The listing builds one solid part. Answer for the finished solid, in the listing's coordinates (mm). Coordinates: 2 decimals unless noted, no trailing zeros.
(1) For a pull along Y with two mould halves and no side action, classify faces 1 (the cylindrical face through (1.359, -1.683, 49.002)), 2 (the flat face through (0, 0, 0)) as +Y half, -Y half, draft (parallel to the pull), parting line (faces both ways), or undercut.
(2) Given P1, Ø4, axis at x = -9, z = 27.5, coming from the +Y side; P2, Ø1.6, axis at x = -1.905, y = -2.54, coming from the +Z side; P3, Ø1.5, axis at y = 18, z = 10.5, coming from the +X side, each flat-ended and moving along its own axis, determine where each tip first touches the part or whether it passes through.
(3) Straight lines are drawn through the part: line 1 (X direction, y = -2.54, z = 49); line 2 (X direction, y = -2, z = 48); line 3 (Y direction, x = 17, z = 12). For each, find the intervals that lie inside material, in ascending order.
from build123d import *

# Parameters (mm, degrees)
F4_D     = 2.032
F4_DEPTH = 3.81
F4_START = 13.0290755
F4_TIP   = 0.6104743889
F5_DEPTH = 17.78


with BuildPart() as f1:
    # F0 (on Front) → F1 (revolve)
    with BuildSketch(Plane.XZ):
        with BuildLine():
            Line((0, 51.8371127546), (0, 0))
            Line((0, 0), (25.6147161126, 0))
            add(Edge.make_bspline(
                [(25.6147161126, 0), (22.8049212909, 20.5093036404), (9.6490421389, 44.5611330733), (4.4700330506, 51.3505992855), (0, 51.8371127546)],
                knots=[0, 0, 0, 0, 0.6778847742, 1, 1, 1, 1], degree=3))
        make_face()
    revolve(axis=Axis((0, 0, 25.9185563773), (0, 0, 1)))

    # F4
    # its depths count from where the whole tool has entered the part; down to there all is cleared
    with Locations(Plane.XY.offset(63.5)):
        with Locations((-1.905, -2.54), (1.905, -2.54)):
            Hole(F4_D / 2, depth=F4_START)
    with Locations(Plane.XY.offset(63.5).offset(-F4_START)):
        with Locations((-1.905, -2.54), (1.905, -2.54)):
            Hole(F4_D / 2, depth=F4_DEPTH)
            with Locations((0, 0, -(F4_DEPTH + F4_TIP / 2))):  # 118° drill point
                Cone(0, F4_D / 2, F4_TIP, mode=Mode.SUBTRACT)

    # F3 (on offset) → F5 (cut)
    with BuildSketch(Plane.XY.offset(63.5)):
        with BuildLine():
            Line((3.7562806858, -6.35), (-3.8637193142, -6.35))
            ThreePointArc((-3.8637193142, -6.35), (-0.0537193142, -8.035230032), (3.7562806858, -6.35))
        make_face()
    extrude(amount=-F5_DEPTH, mode=Mode.SUBTRACT)


solid = f1.part
Model answer:
1. face 1: undercut
1. face 2: draft
2. P1: stops at y = 16.85
2. P2: stops at z = 46.53
2. P3: stops at x = 16.14
3. line 1: x = -5.33 to -2.92, -0.89 to 0.89, 2.92 to 5.33
3. line 2: x = -6.43 to -2.77, -1.04 to 1.04, 2.77 to 6.43
3. line 3: y = -15.81 to 15.81
